from build123d import *

# Parameters (mm, degrees)
F1_DEPTH = 4
F2_W     = 4.1
F2_H     = 2
F2_W_2   = 2
F2_H_2   = 3.7
F2_W_3   = 4.51
F2_W_4   = 2.255
F2_H_3   = 4.566667
F2_H_4   = 4.566666
F2_W_5   = 2.575
F3_DEPTH = 3.2


with BuildPart() as f1:
    # F0 (on Top) → F1 (new body)
    with BuildSketch(Plane.XY):
        Polygon((-16.875, 22.5), (-6.375, 22.5), (-6.375, 0), (6.375, 0), (6.375, 22.5), (16.875, 22.5), (16.875, 37.5), (-16.875, 37.5), align=None)
    extrude(amount=F1_DEPTH)


with BuildPart() as f3:
    # F2 (on face) → F3 (new body)
    with BuildSketch(Plane.XY.offset(4)):
        with Locations((-11.625, 23.5)):
            Rectangle(F2_W, F2_H)
        with Locations((-15.875, 23.5)):
            Rectangle(F2_W_2, F2_H)
        with Locations((-15.875, 27.55)):
            Rectangle(F2_W_2, F2_H_2)
        with Locations((-15.875, 32.45)):
            Rectangle(F2_W_2, F2_H_2)
        with Locations((-11.42, 36.5)):
            Rectangle(F2_W_3, F2_H)
        with Locations((-5.71, 36.5)):
            Rectangle(F2_W_3, F2_H)
        with Locations((-1.1275, 36.5)):
            Rectangle(F2_W_4, F2_H)
        with Locations((-15.875, 36.5)):
            Rectangle(F2_W_2, F2_H)
        with Locations((-5.375, 17.016666)):
            Rectangle(F2_W_2, F2_H_3)
        with Locations((-5.375, 11.25)):
            Rectangle(F2_W_2, F2_H_4)
        with Locations((-5.375, 5.483333)):
            Rectangle(F2_W_2, F2_H_3)
        with Locations((-5.375, 1)):
            Rectangle(F2_W_2, F2_H)
        with Locations((-1.8875, 1)):
            Rectangle(F2_W_5, F2_H)
        Polygon((-8.375, 22.5), (-6.375, 22.5), (-6.375, 20.5), (-4.375, 20.5), (-4.375, 24.5), (-8.375, 24.5), align=None)
    extrude(amount=-F3_DEPTH)


with BuildPart() as f4_1:
    # F4: instance of F3
    add(f3.part.mirror(Plane.YZ))


with BuildPart() as f1_1:
    add(f1.part)

    # F5: cut F3, F4_1
    add(f3.part, mode=Mode.SUBTRACT)
    add(f4_1.part, mode=Mode.SUBTRACT)


solid = f1_1.part
CAD build for the part. Positions are in the model's coordinates, mm. A direction names the side the tool comes from. Give positions to 0.01 mm unless a question says otherwise; leave off trailing zeros. Write each loop counter-clockwise with the first axis right and the second up, starting at its lowest first coordinate (ties: lowest second). Pieces come first, ordered by that corner, then holes. Notation, with made-up numbers: M 9.25,-10.5 L 28.25,-10.5 A15 cw 28.25,2.5 Z; hole C 21,-39 d8. An arc over 180 degrees is marked long. Put each result on its own line as item: value. Start each with the question number.
(1) Mould opens along X. For faces 5 (the face through (-11.7, 22.5, 0.6)), 6 (the face through (-12, 24, 0.8)), 7 (the face through (4.375, 11, 2)), 8 (the face through (-6, 24.5, 2)) say: +X half, -X half, draft (parallel to the pull), parting line (faces both ways), or undercut.
(2) Probe L1, parallel to Y at x = -4, z = 3.85; L2, parallel to X at y = 15, z = 3.8 (3 decimals); L3, parallel to Y at x = 6.5, z = 1.5. List the from-to ranges inside material, lowest first.
(3) Flat gauge pins, fed straight in: pin 1 Ø1 at (x, y) = (10.5, 32) entering from -Z; pin 2 Ø1.2 at (y, z) = (16.5, 2) entering from +X (3 decimals); pin 3 Ø1.5 at (x, z) = (-10.5, 1.5) entering from -Y; pin 4 Ø1.6 at (x, y) = (11, 36.5) entering from +Z. Where does each tip first touch, or does it go through?
(4) Band-saw the part on C-C, the plane y = 28. Write the cut outline in (x, z) (3 decimals), and give its area (3 significant figures).
(5) Band-saw the part on A-A, the plane x = 5.5. Write the cut outline in (y, z).
(6) Band-saw the part on B-B, the plane y = 9.5. Write the cut outline in (x, z) (3 decimals), and give its area (3 significant figures).
(7) Which spindle directions (+Z, -Z, +X, -X, +Y, -Y) get a long thin tool onto all of the face, cutting with end or side? Do faces 1 (the face through (-5, 13.533, 2)), 2 (the face through (-14.875, 36, 2)), 3 (the face through (-14.875, 23, 2)), 4 (the face through (2, 2, 2)). Say none if no direction does.
(8) Band-saw the part on D-D, the plane x = 0. Write the cut outline in (y, z), and give its area (3 significant figures).
Response values:
1. face 5: draft
1. face 6: undercut
1. face 7: +X half
1. face 8: undercut
2. L1: y = 0 to 35.5
2. L2: x = -4.375 to 4.375
2. L3: y = 24.5 to 35.5
3. pin 1: stops at z = 0
3. pin 2: stops at x = 4.375
3. pin 3: stops at y = 22.5
3. pin 4: stops at z = 0.8
4. outline: M -16.875,0 L 16.875,0 L 16.875,0.8 L 14.875,0.8 L 14.875,4 L -14.875,4 L -14.875,0.8 L -16.875,0.8 Z
4. area: 122 mm2
5. outline: M 0,0 L 37.5,0 L 37.5,0.8 L 35.5,0.8 L 35.5,4 L 24.5,4 L 24.5,0.8 L 20.5,0.8 L 20.5,4 L 19.3,4 L 19.3,0.8 L 14.73,0.8 L 14.73,4 L 13.53,4 L 13.53,0.8 L 8.97,0.8 L 8.97,4 L 7.77,4 L 7.77,0.8 L 3.2,0.8 L 3.2,4 L 2,4 L 2,0.8 L 0,0.8 Z
6. outline: M -6.375,0 L 6.375,0 L 6.375,0.8 L 4.375,0.8 L 4.375,4 L -4.375,4 L -4.375,0.8 L -6.375,0.8 Z
6. area: 38.2 mm2
7. face 1: +Z, -X
7. face 2: +Z, -X, +Y
7. face 3: +Z, -X, -Y
7. face 4: +Z, -Y
8. outline: M 0,0 L 37.5,0 L 37.5,0.8 L 35.5,0.8 L 35.5,4 L 0,4 Z
8. area: 144 mm2
